```python
from build123d import *
from build123d import SkipClean  # not in build123d's __all__

# Parameters (mm, degrees)
F1_DEPTH    = 5
F2_T1_DEPTH = 8.0563067351
F2_T3_DEPTH = 8.3213759835
F2_T5_DEPTH = 8.112494996
F2_T7_DEPTH = 9.1625838734


# Not quite as in the source:
# - a fillet or chamfer that OpenCascade refuses, or shapes differently, is made with other operations: its cross-section is extruded or revolved along the edge and cut away or added


with BuildPart() as f1:
    # F0 (on Front) → F1 (new body)
    with BuildSketch(Plane.XZ):
        with BuildLine():
            Line((0, -1), (0, 0))
            Line((0, 0), (-27.9919262234, 0))
            Line((-27.9919262234, 0), (-27.9746514708, -0.3296219153))
            ThreePointArc((-27.9746514708, -0.3296219153), (-34.3872999356, 3.2616337796), (-35.6319805153, -3.9819805153))
            Line((-35.6319805153, -3.9819805153), (-34.217766953, -2.567766953))
            ThreePointArc((-34.217766953, -2.567766953), (-33.4067085809, 1.5096988313), (-29.95, -0.8))
            Line((-29.95, -0.8), (-29.7665727725, -4.3))
            Line((-29.7665727725, -4.3), (0, -4.3))
            Line((0, -4.3), (0, -3.3))
            ThreePointArc((0, -3.3), (-1.15, -2.15), (0, -1))
        make_face()
        with BuildLine():
            Line((-27.95, -0.8), (-27.9746514708, -0.3296219153))
            ThreePointArc((-27.9746514708, -0.3296219153), (-27.9561670936, -0.5644881969), (-27.95, -0.8))
        make_face(mode=Mode.SUBTRACT)
        with BuildLine():
            ThreePointArc((-27.95, -0.8), (-27.9561670936, -0.5644881969), (-27.9746514708, -0.3296219153))
            Line((-27.9746514708, -0.3296219153), (-27.95, -0.8))
        make_face()
    extrude(amount=F1_DEPTH)

    # F2: fillet of radius 0.7 on 4 edges, made by hand

    # F2_s2 → F2_t1 (cut)
    with BuildSketch(Plane.XZ.offset(-1.5281533676)):
        with BuildLine():
            ThreePointArc((-27.3806648764, 0), (-27.7203230433, -0.0879278395), (-27.9746514708, -0.3296219153))
            Line((-27.9746514708, -0.3296219153), (-27.9919262234, 0))
            Line((-27.9919262234, 0), (-27.3806648764, 0))
        make_face()
    extrude(amount=F2_T1_DEPTH, mode=Mode.SUBTRACT)

    # F2_s4 → F2_t3 (cut)
    with BuildSketch(Plane.XZ.offset(-1.6606879918)):
        with BuildLine():
            ThreePointArc((-29.1022975758, -4.3), (-29.5841457788, -4.1077620597), (-29.8013382501, -3.6366351694))
            Line((-29.8013382501, -3.6366351694), (-29.7665727725, -4.3))
            Line((-29.7665727725, -4.3), (-29.1022975758, -4.3))
        make_face()
    extrude(amount=F2_T3_DEPTH, mode=Mode.SUBTRACT)

    # F2_s6 → F2_t5 (cut)
    with BuildSketch(Plane.XZ.offset(-1.556247498)):
        with BuildLine():
            ThreePointArc((-34.6579402166, -3.0079402166), (-34.4571662087, -2.5899957909), (-34.5616523152, -2.1382542732))
            ThreePointArc((-34.5616523152, -2.1382542732), (-34.4015618745, -2.3625), (-34.217766953, -2.567766953))
            Line((-34.217766953, -2.567766953), (-34.6579402166, -3.0079402166))
        make_face()
    extrude(amount=F2_T5_DEPTH, mode=Mode.SUBTRACT)

    # F2_s8 → F2_t7 (cut)
    with BuildSketch(Plane.XZ.offset(-2.0812919367)):
        with BuildLine():
            ThreePointArc((-36.1636809848, -3.3413723739), (-35.6507485808, -3.6430465403), (-35.0910225292, -3.4410225292))
            Line((-35.0910225292, -3.4410225292), (-35.6319805153, -3.9819805153))
            ThreePointArc((-35.6319805153, -3.9819805153), (-35.9126769383, -3.6739986815), (-36.1636809848, -3.3413723739))
        make_face()
    extrude(amount=F2_T7_DEPTH, mode=Mode.SUBTRACT)

    # F3: F1 across plane


with BuildPart() as f1_1:
    add(f1.part, clean=False)
    with SkipClean():  # cleaning this boolean's faces spoils the solid; the shape is the same uncleaned
        add(f1.part.mirror(Plane.YZ), clean=False)


solid = f1_1.part
```
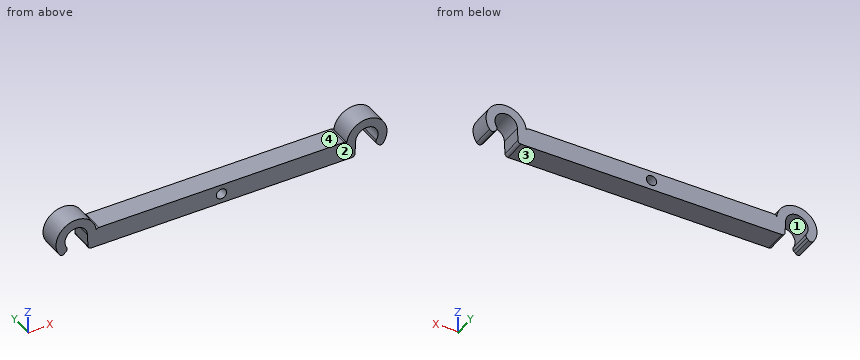
The listing builds one solid part. Answer for the finished solid, in the listing's coordinates (mm). Face numbers are marked on the shaded views. Give positions to 0.01 mm unless a question says otherwise; leave off trailing zeros. Write each loop counter-clockwise with the first axis right and the second up, starting at its lowest first coordinate (ties: lowest second). Pieces come first, ordered by that corner, then holes. Notation, with made-up numbers: (79, 40.25) - (131, 40.25) arc R33 cw to (131, 74.25) - close; hole circle Ø11 at (38.5, 11.25). An arc over 180 degrees is marked (long way). Use one line per item in the form item = value. Start each with the question number.
1) Consider line 1 along X through (y, z) = (-2.5, -2.15); line 2 along X through (y, z) = (-4.25, 1.5); line 3 along X through (y, z) = (-0.95, -3.5). Determine where each line is inside the solid, lowest interval first. Write a range as from..to.
2) A flat-ended cylindrical pin translates along its axis: pin 1 Ø1 at (y, z) = (-1.5, -3.5) entering from +X. Find the tip coordinate at first contact, or state that the pin passes through.
3) Find section C-C on y = -0.95. Determine the outline of the cut face in (x, z).
4) Find section B-B on z = 0.75. Determine the outline of the cut face in (x, y).
5) Find section A-A on x = 0. Determine the outline of the cut face in (y, z).
6) The mould has two halves that part along Z. Classify the marked faces 1, 2, 3 and 4: pulls with the +Z half, pulls with the -Z half, needs draft (parallel to the pull), parting line crosses it, or undercut.
7) Find section D-D on x = -12. Determine the outline of the cut face in (y, z).
Geometry results:
q1.line_1 = -36.74..-34.55, -29.88..-1.15, 1.15..29.88, 34.55..36.74
q1.line_2 = -36.32..-33.43, -31.47..-28.58, 28.58..31.47, 33.43..36.32
q1.line_3 = -36.01..-35.16, -29.81..29.81, 35.16..36.01
q2.pin_1 = 36.38
q3.outline = (-36.16, -3.34) arc R0.7 ccw to (-35.09, -3.44) - (-34.66, -3.01) arc R0.7 ccw to (-34.56, -2.14) arc R2.5 cw (long way) to (-29.95, -0.8) - (-29.8, -3.64) arc R0.7 ccw to (-29.1, -4.3) - (29.1, -4.3) arc R0.7 ccw to (29.8, -3.64) - (29.95, -0.8) arc R2.5 cw (long way) to (34.56, -2.14) arc R0.7 ccw to (34.66, -3.01) - (35.09, -3.44) arc R0.7 ccw to (36.16, -3.34) arc R4.5 ccw (long way) to (27.97, -0.33) arc R0.7 ccw to (27.38, 0) - (-27.38, 0) arc R0.7 ccw to (-27.97, -0.33) arc R4.5 ccw (long way) to start; hole circle Ø2.3 at (0, -2.15)
q4.outline = (-36.67, -5) - (-34.41, -5) - (-34.41, 0) - (-36.67, 0) - close; (-30.49, -5) - (-28.23, -5) - (-28.23, 0) - (-30.49, 0) - close; (28.23, -5) - (30.49, -5) - (30.49, 0) - (28.23, 0) - close; (34.41, -5) - (36.67, -5) - (36.67, 0) - (34.41, 0) - close
q5.outline = (-5, -4.3) - (0, -4.3) - (0, -3.3) - (-5, -3.3) - close; (-5, -1) - (0, -1) - (0, 0) - (-5, 0) - close
q6.face_1 = undercut
q6.face_2 = needs draft
q6.face_3 = pulls with the -Z half
q6.face_4 = pulls with the +Z half
q7.outline = (-5, -4.3) - (0, -4.3) - (0, 0) - (-5, 0) - close
